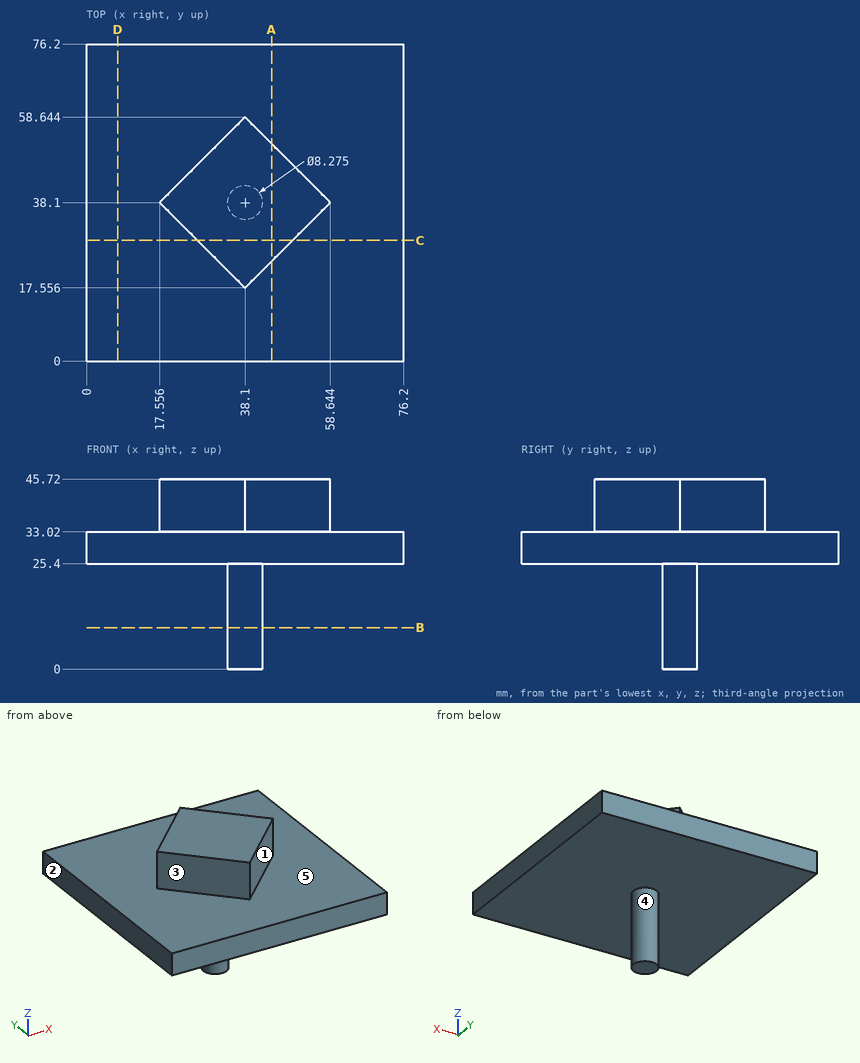
Design review of the part shown in the three views and the two pictorial views. Dimensions are in mm from the part's minimum x, y and z. A direction names the side the tool comes from. Round coordinates to 2 decimals unless told otherwise and drop trailing zeros. Write each loop counter-clockwise with the first axis right and the second up, starting at its lowest first coordinate (ties: lowest second). Pieces come first, ordered by that corner, then holes. Notation, with made-up numbers: (27.5, 22) - (84.5, 22) arc R9 cw to (84.5, 34) - close; hole circle Ø5 at (62.5, 48). An arc over 180 degrees is marked (long way). Answer as CSV lines item,"result". Start each with the question number.
(1) Add section C-C, the plane y = 29. State the section outline as (x, z) points.
(2) Add section A-A, the plane x = 44.5. State the section outline as (y, z) points.
(3) For line 1 (Z direction, x = 41, y = 6.5); line 2 (X direction, y = 54.5, z = 36.5) (1 decimal); line 3 (Y direction, x = 38, z = 13), list the stretches that pass through material, from the lowest coordinate up.
(4) Add section D-D, the plane x = 7.5. State the section outline as (y, z) points.
(5) Machinability: for the marked faces 1, 2, 3, 4 and 5, which of the approach directions +Z, -Z, +X, -X, +Y, -Y give a long, thin tool a straight path to every point of the face, cutting with its end or side? Answer none if there is none.
(6) For pin 1 (5 mm diameter, centred on x = 7.5, y = 67.5, fed in from -Z), flat-tipped, find the tip position at first contact; note if it passes through.
(7) Add section B-B, the plane z = 10. State the section outline as (x, y) points (1 decimal).
From the geometry:
1,outline,"(0, 25.4) - (76.2, 25.4) - (76.2, 33.02) - (49.54, 33.02) - (49.54, 45.72) - (26.66, 45.72) - (26.66, 33.02) - (0, 33.02) - close"
2,outline,"(0, 25.4) - (76.2, 25.4) - (76.2, 33.02) - (52.24, 33.02) - (52.24, 45.72) - (23.96, 45.72) - (23.96, 33.02) - (0, 33.02) - close"
3,line 1,"z = 25.4 to 33.02"
3,line 2,"x = 34 to 42.2"
3,line 3,"y = 33.96 to 42.24"
4,outline,"(0, 25.4) - (76.2, 25.4) - (76.2, 33.02) - (0, 33.02) - close"
5,face 1,"+Z, +X, -Y"
5,face 2,"+Z, -Z, -X, +Y, -Y"
5,face 3,"+Z, -X, -Y"
5,face 4,"-Z"
5,face 5,"+Z"
6,pin 1,"stops at z = 25.4"
7,outline,"circle Ø8.3 at (38.1, 38.1)"
